The model under review builds one solid part; all positions refer to its coordinate system, in mm. Face numbers are marked on the shaded views. A direction names the side the tool comes from. Coordinates: 2 decimals unless noted, no trailing zeros. Order: outer loops, then holes, each group sorted by start corner. A loop starts at its lowest first (then second) coordinate and runs counter-clockwise, first axis right, second up. Notation, with made-up numbers: (41, -16) -> (75, -16) arc R7 cw to (75, -3) -> close; hole circle Ø6 at (31, 57.25). An arc over 180 degrees is marked (long way). Put each result on its own line as item: value.
from build123d import *

# Parameters (mm, degrees)
MODEL_R                 = 1.5
SALIENTE_EXTRUIR1_DEPTH = 3


with BuildPart() as part:
    # Model → Saliente-Extruir1 (new body)
    with BuildSketch(Plane.XY):
        with BuildLine():
            Line((202.97316991, 160.056557042), (202.97316991, 182.556557042))
            ThreePointArc((202.97316991, 182.556557042), (207.47316991, 187.056557042), (211.97316991, 182.556557042))
            Line((211.97316991, 182.556557042), (211.97316991, 160.056557042))
            Line((211.97316991, 160.056557042), (202.97316991, 160.056557042))
        make_face()
        with Locations((207.47316991, 173.556557042)):
            Circle(MODEL_R, mode=Mode.SUBTRACT)
        with Locations((207.47316991, 182.556557042)):
            Circle(MODEL_R, mode=Mode.SUBTRACT)
        with BuildLine():
            Line((205.84816991, 162.056557042), (205.84816991, 167.056557042))
            ThreePointArc((205.84816991, 167.056557042), (206.067839825, 167.586887128), (206.59816991, 167.806557042))
            Line((206.59816991, 167.806557042), (208.34816991, 167.806557042))
            ThreePointArc((208.34816991, 167.806557042), (208.878499996, 167.586887128), (209.09816991, 167.056557042))
            Line((209.09816991, 167.056557042), (209.09816991, 162.056557042))
            ThreePointArc((209.09816991, 162.056557042), (208.878499996, 161.526226956), (208.34816991, 161.306557042))
            Line((208.34816991, 161.306557042), (206.59816991, 161.306557042))
            ThreePointArc((206.59816991, 161.306557042), (206.067839825, 161.526226956), (205.84816991, 162.056557042))
        make_face(mode=Mode.SUBTRACT)
    extrude(amount=SALIENTE_EXTRUIR1_DEPTH)


solid = part.part
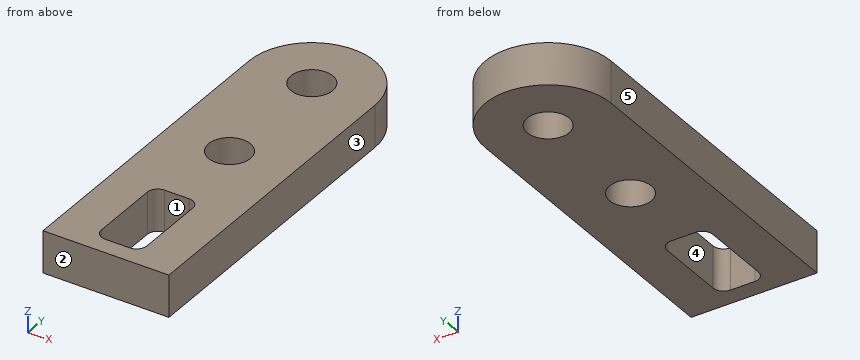
Item 1: Consider section B-B on x = 207.25. Write out the cut boundary in (y, z).
Answers below:
outline: (160.06, 0) -> (161.31, 0) -> (161.31, 3) -> (160.06, 3) -> close; (167.81, 0) -> (172.07, 0) -> (172.07, 3) -> (167.81, 3) -> close; (175.04, 0) -> (181.07, 0) -> (181.07, 3) -> (175.04, 3) -> close; (184.04, 0) -> (187.05, 0) -> (187.05, 3) -> (184.04, 3) -> close
Item 2: Consider section C-C on z = 2.4. Write out the cut boundary in (x, y).
Answers below:
outline: (202.97, 160.06) -> (211.97, 160.06) -> (211.97, 182.56) arc R4.5 ccw to (202.97, 182.56) -> close; hole (205.85, 162.06) arc R0.75 ccw to (206.6, 161.31) -> (208.35, 161.31) arc R0.75 ccw to (209.1, 162.06) -> (209.1, 167.06) arc R0.75 ccw to (208.35, 167.81) -> (206.6, 167.81) arc R0.75 ccw to (205.85, 167.06) -> close; hole circle Ø3 at (207.47, 173.56); hole circle Ø3 at (207.47, 182.56)
Item 3: For line 1 (X direction, y = 164.75, z = 0.7); line 2 (Y direction, x = 208.5, z = 2.7); line 3 (Y direction, x = 208.75, z = 0.2), list the stretches that pass through material, from the lowest coordinate up. Write a range as from..to.
Answers below:
line 1: 202.97..205.85, 209.1..211.97
line 2: 160.06..161.32, 167.79..172.46, 174.65..181.46, 183.65..186.94
line 3: 160.06..161.42, 167.69..172.77, 174.34..181.77, 183.34..186.87
Item 4: Consider section D-D on y = 174.25. Write out the cut boundary in (x, z), and give its area (3 significant figures).
Answers below:
outline: (202.97, 0) -> (206.14, 0) -> (206.14, 3) -> (202.97, 3) -> close; (208.8, 0) -> (211.97, 0) -> (211.97, 3) -> (208.8, 3) -> close
area: 19.0 mm^2
Item 5: Consider section A-A on y = 165. Write out the cut boundary in (x, z), and give its area (4 significant figures).
Answers below:
outline: (202.97, 0) -> (205.85, 0) -> (205.85, 3) -> (202.97, 3) -> close; (209.1, 0) -> (211.97, 0) -> (211.97, 3) -> (209.1, 3) -> close
area: 17.25 mm^2
Item 6: Mouldability with a two-part tool opening along X and no side actions: class the marked faces 1, 2 and 3 as +X half, -X half, draft (parallel to the pull), parting line (faces both ways), or undercut.
Answers below:
face 1: undercut
face 2: draft
face 3: +X half
Item 7: For the marked faces 4 and 5, list the 3-axis set-ups (+Z, -Z, +X, -X, +Y, -Y) from which the entire face can be reached by the end or side of a thin tool; tool diameter is ignored.
Answers below:
face 4: +Z, -Z
face 5: +Z, -Z, -X, +Y, -Y
